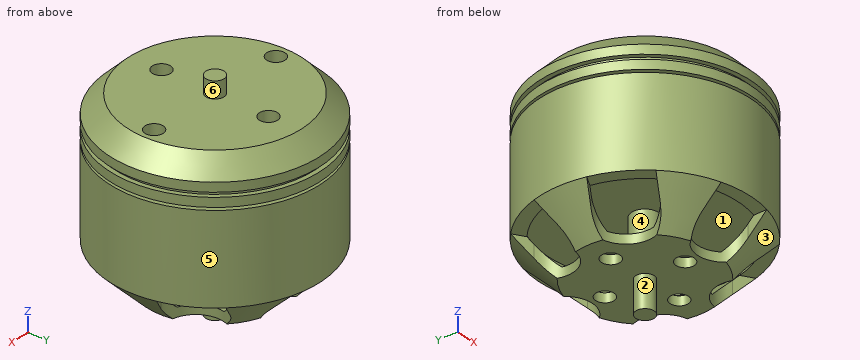
from build123d import *

# Parameters (mm, degrees)
SKETCH3_R          = 1
CUT_EXTRUDE1_DEPTH = 4
SKETCH4_R          = 1
CUT_EXTRUDE2_DEPTH = 3


with BuildPart() as part:
    # Sketch2 → Revolve1 (revolve)
    with BuildSketch(Plane(origin=(0, 0, 0), x_dir=(1, 0, 0), z_dir=(0, 1, 0))):
        Polygon((0, 20.711668775), (0, 0), (0, -3.088331225), (1, -3.088331225), (1, -1.288331225), (9.5, -1.288331225), (11.5, 0.711668775), (11.5, 1.711668775), (11, 1.711668775), (11, 2.211668775), (11.5, 2.211668775), (11.5, 3.211668775), (9.5, 3.211668775), (9.5, 3.511668775), (11.5, 3.511668775), (11.5, 13.211668775), (7.5, 17.211668775), (1, 17.211668775), (1, 20.711668775), align=None)
        Polygon((2.454698557, 16.211668775), (2.454698557, 15.211668775), (1.454698557, 15.211668775), (1.454698557, 11.092814322), (10.5, 11.092814322), (10.5, 12.797455213), (7.085786438, 16.211668775), align=None, mode=Mode.SUBTRACT)
    revolve(axis=Axis((0, 0, -20.711668775), (0, 0, 1)))

    # Sketch3 → Cut-Extrude1 (cut)
    with BuildSketch(Plane(origin=(0, 0, -17.211668775), x_dir=(-1, 0, 0), z_dir=(0, 0, -1))):
        with Locations((0, 4.5)):
            Circle(SKETCH3_R)
        with Locations((4.5, 0)):
            Circle(SKETCH3_R)
        with Locations((0, -4.5)):
            Circle(SKETCH3_R)
        with Locations((-4.5, 0)):
            Circle(SKETCH3_R)
        with BuildLine():
            Line((-3, 9), (-3, 16.651953035))
            Line((-3, 16.651953035), (3, 16.651953035))
            Line((3, 16.651953035), (3, 9))
            ThreePointArc((3, 9), (0, 6), (-3, 9))
        make_face()
        with BuildLine():
            Line((15.921014351, 5.727900306), (9.294228634, 1.901923789))
            ThreePointArc((9.294228634, 1.901923789), (5.196152423, 3), (6.294228634, 7.098076211))
            Line((6.294228634, 7.098076211), (12.921014351, 10.924052729))
            Line((12.921014351, 10.924052729), (15.921014351, 5.727900306))
        make_face()
        with BuildLine():
            Line((12.921014351, -10.924052729), (6.294228634, -7.098076211))
            ThreePointArc((6.294228634, -7.098076211), (5.196152423, -3), (9.294228634, -1.901923789))
            Line((9.294228634, -1.901923789), (15.921014351, -5.727900306))
            Line((15.921014351, -5.727900306), (12.921014351, -10.924052729))
        make_face()
        with BuildLine():
            Line((-3, -16.651953035), (-3, -9))
            ThreePointArc((-3, -9), (0, -6), (3, -9))
            Line((3, -9), (3, -16.651953035))
            Line((3, -16.651953035), (-3, -16.651953035))
        make_face()
        with BuildLine():
            Line((-15.921014351, -5.727900306), (-9.294228634, -1.901923789))
            ThreePointArc((-9.294228634, -1.901923789), (-5.196152423, -3), (-6.294228634, -7.098076211))
            Line((-6.294228634, -7.098076211), (-12.921014351, -10.924052729))
            Line((-12.921014351, -10.924052729), (-15.921014351, -5.727900306))
        make_face()
        with BuildLine():
            Line((-12.921014351, 10.924052729), (-6.294228634, 7.098076211))
            ThreePointArc((-6.294228634, 7.098076211), (-5.196152423, 3), (-9.294228634, 1.901923789))
            Line((-9.294228634, 1.901923789), (-15.921014351, 5.727900306))
            Line((-15.921014351, 5.727900306), (-12.921014351, 10.924052729))
        make_face()
    extrude(amount=-CUT_EXTRUDE1_DEPTH, mode=Mode.SUBTRACT)

    # Sketch4 → Cut-Extrude2 (cut)
    with BuildSketch(Plane.XY.offset(1.288331225)):
        with Locations((0, 6)):
            Circle(SKETCH4_R)
        with Locations((0, -6)):
            Circle(SKETCH4_R)
        with Locations((8, 0)):
            Circle(SKETCH4_R)
        with Locations((-8, 0)):
            Circle(SKETCH4_R)
    extrude(amount=-CUT_EXTRUDE2_DEPTH, mode=Mode.SUBTRACT)


solid = part.part
The model under review builds one solid part; all positions refer to its coordinate system, in mm. Face numbers are marked on the shaded views. A direction names the side the tool comes from. Give positions to 0.01 mm unless a question says otherwise; leave off trailing zeros. Order: outer loops, then holes, each group sorted by start corner. A loop starts at its lowest first (then second) coordinate and runs counter-clockwise, first axis right, second up. Notation, with made-up numbers: M 22.25,-9.5 L 45.25,-9.5 A32 ccw 45.25,18.5 Z; hole C -8.5,38 d11. An arc over 180 degrees is marked long. Use one line per item in the form item = value. Start each with the question number.
Item 1: To check wall thickness, follow line 1 along Y through (x, z) = (0, -16.45); line 2 along Z through (x, y) = (4.5, 5); line 3 along Z through (x, y) = (-6.5, -8). State the ranges of each line that lie inside material, in increasing order. Write a range as from..to.
Item 2: We need section A-A on z = -7.25. Give the boundary of the cut face in (x, y), plus the area to 3 significant figures.
Item 3: We need section B-B on x = 0. Give the number of separate pieces and of enclosed holes in the cut face, plus the area to 3 significant figures.
Item 4: For the marked faces 4, 5 and 6, list the 3-axis set-ups (+Z, -Z, +X, -X, +Y, -Y) from which the entire face can be reached by the end or side of a thin tool; tool diameter is ignored.
Item 5: Insertion check: pin 1 Ø1.5 at (y, z) = (1.5, -17.5) entering from -X; pin 2 Ø1.8 at (x, y) = (0, 4.5) entering from -Z; pin 3 Ø4 at (x, z) = (3.5, -14) entering from +Y; pin 4 Ø12 at (x, y) = (-2, -0.5) entering from -Z. Each pin has a flat end and moves straight along its axis. Give the tip position at first contact, or say it passes through.
Item 6: The part is to be moulded in two halves that separate along Z. For the marked faces 1, 2 and 3, say which applies: pulls with the +Z half, pulls with the -Z half, needs draft (parallel to the pull), parting line crosses it, or undercut.
Completed:
q1.line_1 = -6..-5.5, -3.5..3.5, 5.5..6
q1.line_2 = -17.21..-16.21, -11.09..1.29
q1.line_3 = -14.4..-12.99, -11.09..-3.51, -3.21..0.48
q2.outline = C 0,0 d23
q2.area = 415 mm²
q3.separate_pieces = 3
q3.enclosed_holes = 0
q3.area = 307 mm²
q4.face_4 = none
q4.face_5 = +Z, -Z
q4.face_6 = +Z
q5.pin_1 = -7.83
q5.pin_2 = -11.09
q5.pin_3 = 11.38
q5.pin_4 = -20.71
q6.face_1 = undercut
q6.face_2 = needs draft
q6.face_3 = pulls with the -Z half
